Verification items for this drawing (mm, ordinates from the low corner). A direction names the side the tool comes from. Give positions to 0.01 mm unless a question says otherwise; leave off trailing zeros. Write each loop counter-clockwise with the first axis right and the second up, starting at its lowest first coordinate (ties: lowest second). Pieces come first, ordered by that corner, then holes. Notation, with made-up numbers: (-23, -28.75) -> (-7, -28.75) arc R22 cw to (-7, 3.25) -> close; hole circle Ø3 at (42.25, 13). An arc over 180 degrees is marked (long way). One line per item, written item: value.
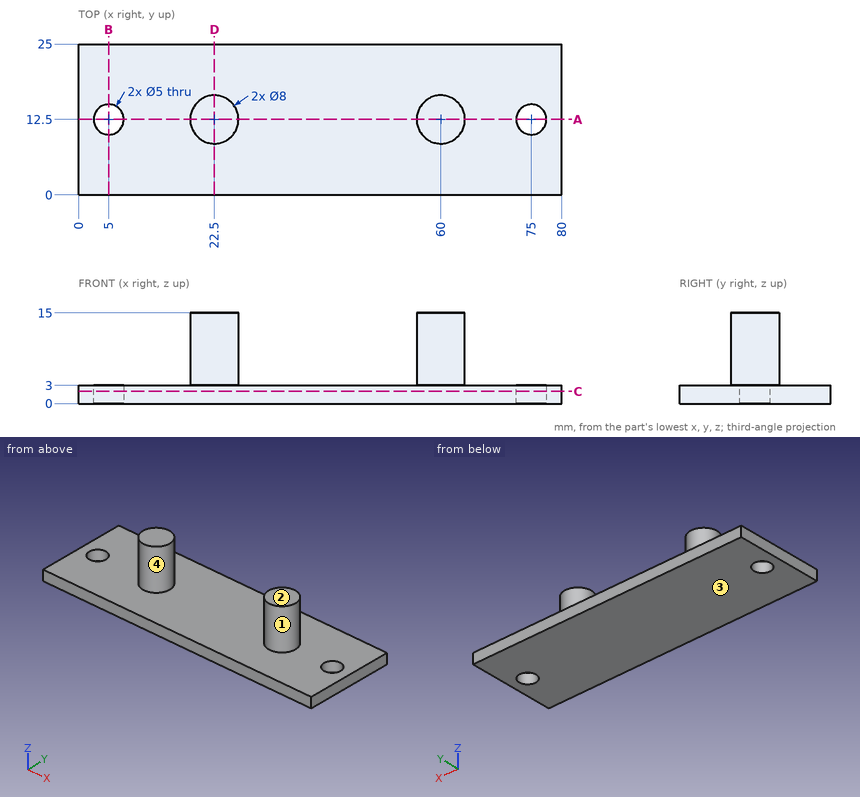
1) Mould release check, pull along X, two halves, no side actions. Record for the marked faces 3 and 4: released by +X, released by -X, zero draft, split by the parting line, or undercut.
Verdict:
face 3: zero draft
face 4: undercut
2) Sectioned sample at B-B on x = 5. Record the cut outline in (y, z), plus the area to 3 significant figures.
Verdict:
outline: (0, 0) -> (10, 0) -> (10, 3) -> (0, 3) -> close; (15, 0) -> (25, 0) -> (25, 3) -> (15, 3) -> close
area: 60.0 mm^2
3) Tool access check on the marked faces 1 and 2. Record the directions out of +Z, -Z, +X, -X, +Y, -Y that give a thin tool (end or side, any length) a straight path to the whole face; none if there is none.
Verdict:
face 1: +Z
face 2: +Z, +X, -X, +Y, -Y
4) Sectioned sample at D-D on x = 22.5. Record the cut outline in (y, z).
Verdict:
outline: (0, 0) -> (25, 0) -> (25, 3) -> (16.5, 3) -> (16.5, 15) -> (8.5, 15) -> (8.5, 3) -> (0, 3) -> close
5) Sectioned sample at C-C on z = 2. Record the cut outline in (x, y).
Verdict:
outline: (0, 0) -> (80, 0) -> (80, 25) -> (0, 25) -> close; hole circle Ø5 at (5, 12.5); hole circle Ø5 at (75, 12.5)
6) Depth check by flat-ended pin: pin 1 Ø3 at (x, y) = (41, 13.5) entering from +Z; pin 2 Ø6 at (x, y) = (75, 12.5) entering from -Z; pin 3 Ø3 at (y, z) = (21, 6) entering from +X; pin 4 Ø1.5 at (y, z) = (14, 11.5) entering from +X. Enter the tip coordinate at first touch or a pass-through.
Verdict:
pin 1: z = 3
pin 2: z = 0
pin 3: through
pin 4: x = 63.93
7) Sectioned sample at A-A on y = 12.5. Record the cut outline in (x, z).
Verdict:
outline: (0, 0) -> (2.5, 0) -> (2.5, 3) -> (0, 3) -> close; (7.5, 0) -> (72.5, 0) -> (72.5, 3) -> (64, 3) -> (64, 15) -> (56, 15) -> (56, 3) -> (26.5, 3) -> (26.5, 15) -> (18.5, 15) -> (18.5, 3) -> (7.5, 3) -> close; (77.5, 0) -> (80, 0) -> (80, 3) -> (77.5, 3) -> close
8) Scan lines: probe 1 along Z at (x, y) = (51, 19.25); probe 2 along Y at (x, z) = (5, 1.6); probe 3 along Y at (x, z) = (58, 13.75). Record each from-to range of solid material in increasing order.
Verdict:
probe 1: 0 to 3
probe 2: 0 to 10, 15 to 25
probe 3: 9.04 to 15.96
